```python
from build123d import *

# Parameters (mm, degrees)
SKETCH1_R           = 1.6
BOSS_EXTRUDE1_DEPTH = 5.08
SHELL1_START        = 2.54
SHELL1_DEPTH        = 2.54
CUT_EXTRUDE1_DEPTH  = 2.54


# Read off the part's stored shape, not the designer's step: Shell1
with BuildPart() as part:
    # Sketch1 → Boss-Extrude1 (new body)
    with BuildSketch(Plane(origin=(0, 0, 0), x_dir=(1, 0, 0), z_dir=(0, 1, 0))):
        Polygon((-5.08, -6.35), (5.08, -6.35), (5.08, -19.05), (26.67, -19.05), (26.67, 19.05), (-26.67, 19.05), (-26.67, -19.05), (-5.08, -19.05), align=None)
        with Locations(Location((12.065, -6.35, 0), (0, 0, 270))):
            Circle(SKETCH1_R, mode=Mode.SUBTRACT)
        with Locations(Location((-22.86, 15.24, 0), (0, 0, 270))):
            Circle(SKETCH1_R, mode=Mode.SUBTRACT)
        with Locations(Location((16.764, -1.905, 0), (0, 0, 270))):
            Circle(SKETCH1_R, mode=Mode.SUBTRACT)
        with Locations(Location((-22.86, 7.62, 0), (0, 0, 270))):
            Circle(SKETCH1_R, mode=Mode.SUBTRACT)
        with Locations(Location((22.86, 15.24, 0), (0, 0, 270))):
            Circle(SKETCH1_R, mode=Mode.SUBTRACT)
    extrude(amount=BOSS_EXTRUDE1_DEPTH)

    # Shell1 outline → Shell1 (cut)
    with BuildSketch(Plane(origin=(0, 0, 0), x_dir=(1, 0, 0), z_dir=(0, 1, 0)).offset(SHELL1_START)):
        with BuildLine():
            Line((-7.62, -16.51), (-7.62, -3.81))
            Line((-7.62, -3.81), (7.62, -3.81))
            Line((7.62, -3.81), (7.62, -16.51))
            Line((7.62, -16.51), (24.13, -16.51))
            Line((24.13, -16.51), (24.13, 11.299606619))
            ThreePointArc((24.13, 11.299606619), (19.932577926, 12.312577926), (18.919606619, 16.51))
            Line((18.919606619, 16.51), (-18.919606619, 16.51))
            ThreePointArc((-18.919606619, 16.51), (-19.094323259, 13.519744587), (-21.240277802, 11.43))
            ThreePointArc((-21.240277802, 11.43), (-18.980860173, 6.173668709), (-24.13, 3.679606619))
            Line((-24.13, 3.679606619), (-24.13, -16.51))
            Line((-24.13, -16.51), (-7.62, -16.51))
        make_face()
        with BuildLine():
            ThreePointArc((12.638391662, -2.249899757), (19.771579246, 0.940007395), (16.190608338, -6.005100243))
            ThreePointArc((16.190608338, -6.005100243), (9.057420754, -9.195007395), (12.638391662, -2.249899757))
        make_face(mode=Mode.SUBTRACT)
    extrude(amount=SHELL1_DEPTH, mode=Mode.SUBTRACT)

    # Sketch8 → Cut-Extrude1 (cut)
    with BuildSketch(Plane(origin=(0, 5.08, 0), x_dir=(1, 0, 0), z_dir=(0, 1, 0))):
        Polygon((-19.8577786, 15.24), (-21.3588893, 17.84), (-24.3611107, 17.84), (-25.8622214, 15.24), (-24.3611107, 12.64), (-21.3588893, 12.64), align=None)
        Polygon((25.8622214, 15.24), (24.3611107, 17.84), (21.3588893, 17.84), (19.8577786, 15.24), (21.3588893, 12.64), (24.3611107, 12.64), align=None)
        Polygon((15.0672214, -6.35), (13.5661107, -3.75), (10.5638893, -3.75), (9.0627786, -6.35), (10.5638893, -8.95), (13.5661107, -8.95), align=None)
    extrude(amount=-CUT_EXTRUDE1_DEPTH, mode=Mode.SUBTRACT)


solid = part.part
```
The model under review builds one solid part; all positions refer to its coordinate system, in mm. A direction names the side the tool comes from. Coordinates: 2 decimals unless noted, no trailing zeros. Write each loop counter-clockwise with the first axis right and the second up, starting at its lowest first coordinate (ties: lowest second). Pieces come first, ordered by that corner, then holes.
1) Clearance check with flat-ended pins moving along their axes: pin 1 Ø1.6 at (x, z) = (11.5, 7.5) entering from +Y; pin 2 Ø3 at (x, z) = (16.764, 1.905) entering from +Y; pin 3 Ø3 at (x, y) = (-3, 1.5) entering from +Z. State where each tip first meets the part, or that it passes through.
2) The part is to be moulded in two halves that separate along X. For faces 4 (the face through (16, 3, 19.05)), 5 (the face through (24.13, 4, 3)), 6 (the face through (-26.67, 3, 0)), say which applies: pulls with the +X half, pulls with the -X half, needs draft (parallel to the pull), parting line crosses it, or undercut.
3) We need section D-D on x = 4.5. State the section outline as (y, z) points, then the cut area to 3 significant figures.
4) We need section B-B on x = -22.86. State the section outline as (y, z) points.
5) Machinability: for faces 1 (the face through (0, 3, 6.35)), 2 (the face through (16, 4, 16.51)), 3 (the face through (0, 3, -19.05)), which of the approach directions +Z, -Z, +X, -X, +Y, -Y give a long, thin tool a straight path to every point of the face, cutting with its end or side? Answer none if there is none.
6) To check wall thickness, follow probe 1 along X at (y, z) = (1.15, -7.62); probe 2 along Z at (x, y) = (1.5, 3.75); probe 3 along Z at (x, y) = (-16.5, 3.65). State the ranges of each line that lie inside material, in increasing order.
7) We need section C-C on x = 22.86. State the section outline as (y, z) points, then the cut area to 3 significant figures.
8) We need section A-A on z = -7.62. State the section outline as (x, y) points.
Answer list:
1. pin 1: stops at y = 2.54
1. pin 2: passes through
1. pin 3: stops at z = 6.35
2. face 4: needs draft
2. face 5: undercut
2. face 6: pulls with the -X half
3. outline: (0, -19.05) - (5.08, -19.05) - (5.08, -16.51) - (2.54, -16.51) - (2.54, 3.81) - (5.08, 3.81) - (5.08, 6.35) - (0, 6.35) - close
3. area: 77.4 mm2
4. outline: (0, -19.05) - (5.08, -19.05) - (5.08, -17.84) - (2.54, -17.84) - (2.54, -16.84) - (0, -16.84) - close; (0, -13.64) - (2.54, -13.64) - (2.54, -12.64) - (5.08, -12.64) - (5.08, -9.22) - (0, -9.22) - close; (0, -6.02) - (5.08, -6.02) - (5.08, -3.48) - (2.54, -3.48) - (2.54, 16.51) - (5.08, 16.51) - (5.08, 19.05) - (0, 19.05) - close
5. face 1: +Z, +Y, -Y
5. face 2: +Y
5. face 3: -Z, +X, -X, +Y, -Y
6. probe 1: x = -26.67 to -24.46, -21.26 to 26.67
6. probe 2: z = -19.05 to -16.51, 3.81 to 6.35
6. probe 3: z = -19.05 to -16.51, 16.51 to 19.05
7. outline: (0, -19.05) - (5.08, -19.05) - (5.08, -17.84) - (2.54, -17.84) - (2.54, -16.84) - (0, -16.84) - close; (0, -13.64) - (2.54, -13.64) - (2.54, -12.64) - (5.08, -12.64) - (5.08, -11.1) - (2.54, -11.1) - (2.54, 16.51) - (5.08, 16.51) - (5.08, 19.05) - (0, 19.05) - close
7. area: 102 mm2
8. outline: (-26.67, 0) - (-24.46, 0) - (-24.46, 5.08) - (-26.67, 5.08) - close; (-21.26, 0) - (26.67, 0) - (26.67, 5.08) - (24.13, 5.08) - (24.13, 2.54) - (-18.72, 2.54) - (-18.72, 5.08) - (-21.26, 5.08) - close
